Check sheet for the modelled part. Datum: model origin and axes. Units: mm. A direction names the side the tool comes from. Give positions to 0.01 mm unless a question says otherwise; leave off trailing zeros. Loops run counter-clockwise (first coordinate to the right, second up) from the corner with the lowest first, then second, coordinate; pieces in that order, holes last. Notation, with made-up numbers: (78.25, 47) -> (94.25, 47) arc R11 cw to (94.25, 58) -> close; hole circle Ø8 at (65, 84.5). An arc over 180 degrees is marked (long way). Write each question's results on one line, items separated by ' | '. Start each with the question number.
Item 1: Scan lines: line 1 along Z through (x, y) = (0.75, -0.75); line 2 along Z through (x, y) = (3.5, 0); line 3 along X through (y, z) = (-0.5, 31). Record each from-to range of solid material in increasing order.
Item 2: Cross-section at A-A on x = 0. Enter the section's corners in (y, z), then the cut area to 3 significant figures.
Item 3: Cross-section at B-B on z = 28. Enter the section's corners in (x, y).
Item 4: Mould release check, pull along X, two halves, no side actions. Record for faces 4 (the face through (0, 0, 2.6)), 5 (the face through (2.285, -3.584, 2.465)), 6 (the face through (0, 0, 35)): pulls with the +X half, pulls with the -X half, needs draft (parallel to the pull), parting line crosses it, or undercut.
Item 5: Cross-section at C-C on y = -0.75. Enter the section's corners in (x, z).
Item 6: Cross-section at D-D on x = 3. Enter the section's corners in (y, z), then the cut area to 3 significant figures.
Item 7: Gauge pin test, flat ends, axial feed: pin 1 Ø4 at (y, z) = (1, 25) entering from -X; pin 2 Ø3 at (x, z) = (-2, 26) entering from +Y; pin 3 Ø3 at (y, z) = (2, 17.5) entering from +X. Record the tip position at first contact, or that the pin passes through.
Item 8: Access from +Z, -Z, +X, -X, +Y, -Y to the whole of each face (thin tool, end or side, straight path). Record for faces 1 (the face through (-1.68, -0.99, 1.28)), 2 (the face through (2, -1, 0)), 3 (the face through (-0.54, 2.44, 19.79)).
Solid Edge part; units mm, degrees
sketch "Sketch1" plane through (0, 0, 0) normal (0, 0, 1) x (1, 0, 0)
  circle A0 centre (0, 0) radius 4.25
extrude "Protrusion1" add sketch "Sketch1" along normal blind 5
sketch "Sketch2" plane through (0, 0, 5) normal (0, 0, 1) x (1, 0, 0)
  circle A0 centre (0, 0) radius 2.5
extrude "ExtrudedProtrusion_2" add sketch "Sketch2" along normal blind 30
sketch "Sketch3" plane through (0, 0, 0) normal (0, 0, -1) x (-1, 0, 0)
  line L0 (2.25, 0) -> (1.125, 1.9486)
  line L1 (1.125, 1.9486) -> (-1.125, 1.9486)
  line L2 (-1.125, 1.9486) -> (-2.25, 0)
  line L3 (-2.25, 0) -> (-1.125, -1.9486)
  line L4 (-1.125, -1.9486) -> (1.125, -1.9486)
  line L5 (1.125, -1.9486) -> (2.25, 0)
extrude "ExtrudedCutout_1" cut sketch "Sketch3" against normal blind 2.6
properties material "Stainless steel"
Answer sheet:
1) line 1: z = 2.6 to 35 | line 2: z = 0 to 5 | line 3: x = -2.45 to 2.45
2) outline: (-4.25, 0) -> (-1.95, 0) -> (-1.95, 2.6) -> (1.95, 2.6) -> (1.95, 0) -> (4.25, 0) -> (4.25, 5) -> (2.5, 5) -> (2.5, 35) -> (-2.5, 35) -> (-2.5, 5) -> (-4.25, 5) -> close | area: 182 mm²
3) outline: circle Ø5 at (0, 0)
4) face 4: undercut | face 5: parting line crosses it | face 6: needs draft
5) outline: (-4.18, 0) -> (-1.82, 0) -> (-1.82, 2.6) -> (1.82, 2.6) -> (1.82, 0) -> (4.18, 0) -> (4.18, 5) -> (2.38, 5) -> (2.38, 35) -> (-2.38, 35) -> (-2.38, 5) -> (-4.18, 5) -> close
6) outline: (-3.01, 0) -> (3.01, 0) -> (3.01, 5) -> (-3.01, 5) -> close | area: 30.1 mm²
7) pin 1: stops at x = -2.5 | pin 2: stops at y = 2.45 | pin 3: stops at x = 2.45
8) face 1: -Z | face 2: -Z, +X, -X, +Y, -Y | face 3: +Z
